from build123d import *

# Parameters (mm, degrees)
F0_R     = 19.4437
F1_DEPTH = 9.652
F2_SIZE  = 0.381
F3_R     = 0.254


with BuildPart() as f1:
    # F0 (on Front) → F1 (new body)
    with BuildSketch(Plane.XZ):
        with BuildLine():
            Line((-22.352, 17.802211), (-22.352, -17.802211))
            ThreePointArc((-22.352, -17.802211), (28.575, 0), (-22.352, 17.802211))
        make_face()
        Circle(F0_R, mode=Mode.SUBTRACT)
    extrude(amount=F1_DEPTH)

    # F2
    f2_edges = [f1.edges().sort_by_distance(p)[0] for p in [
        (-19.4437, -9.652, 0),
        (-19.4437, 0, 0),
    ]]
    chamfer(f2_edges, length=F2_SIZE)

    # F3
    f3_edges = [f1.edges().sort_by_distance(p)[0] for p in [
        (28.575, -9.652, 0),
        (28.575, 0, 0),
    ]]
    fillet(f3_edges, radius=F3_R)


solid = f1.part
The model under review builds one solid part; all positions refer to its coordinate system, in mm. Round coordinates to 2 decimals unless told otherwise and drop trailing zeros. Write each loop counter-clockwise with the first axis right and the second up, starting at its lowest first coordinate (ties: lowest second). Pieces come first, ordered by that corner, then holes. Notation, with made-up numbers: (41, 7.25) - (51, 7.25) arc R25 cw to (51, 22.25) - close; hole circle Ø6 at (-4, 14.5). An arc over 180 degrees is marked (long way). One line per item, written item: value. Start each with the question number.
1. Clearance check with flat-ended pins moving along their axes: P1, Ø5, axis at x = 14, z = -18, coming from the +Y side; P2, Ø4, axis at x = 22.5, y = -5.5, coming from the +Z side; P3, Ø1.5, axis at x = -3, y = -4.5, coming from the -Z side. State where each tip first meets the part, or that it passes through.
2. Consider section A-A on z = 0. Write out the cut boundary in (x, y) (3 decimals), and give its area (3 significant figures).
3. The part is to be moulded in two halves that separate along X. For faces 1 (the face through (-4.22, -4.76, -18.98)), 2 (the face through (-22.352, -5, 0)), 3 (the face through (20, 0, 7)), 4 (the face through (28.558, -4.762, -0.988)), say which applies: released by +X, released by -X, zero draft, split by the parting line, or undercut.
4. Consider section B-B on y = -1.75. Write out the cut boundary in (x, z) (3 decimals).
5. To check wall thickness, follow L1, parallel to Z at x = 0, y = -6.5 (3 decimals); L2, parallel to Z at x = -5, y = -1.75; L3, parallel to X at y = -1.25, z = 2. State the ranges of each line that lie inside material, in increasing order. Write a range as from..to.
Checks:
1. P1: stops at y = 0
1. P2: stops at z = 19.91
1. P3: stops at z = -28.49
2. outline: (-22.352, -9.652) - (-19.825, -9.652) - (-19.444, -9.271) - (-19.444, -0.381) - (-19.825, 0) - (-22.352, 0) - close; (19.444, -9.271) - (19.825, -9.652) - (28.321, -9.652) arc R0.254 ccw to (28.575, -9.398) - (28.575, -0.254) arc R0.254 ccw to (28.321, 0) - (19.825, 0) - (19.444, -0.381) - close
2. area: 116 mm^2
3. face 1: undercut
3. face 2: released by -X
3. face 3: zero draft
3. face 4: split by the parting line
4. outline: (-22.352, -17.802) arc R28.575 ccw (long way) to (-22.352, 17.802) - close; hole circle Ø38.887 at (0, 0)
5. L1: z = -28.575..-19.444, 19.444..28.575
5. L2: z = -28.13..-18.79, 18.79..28.13
5. L3: x = -22.35..-19.34, 19.34..28.5
